Design review of the part built by this model. Coordinates are the model's own, in mm. A direction names the side the tool comes from. Give positions to 0.01 mm unless a question says otherwise; leave off trailing zeros. Loops run counter-clockwise (first coordinate to the right, second up) from the corner with the lowest first, then second, coordinate; pieces in that order, holes last. Notation, with made-up numbers: M -31,-3.5 L 19,-3.5 A23 cw 19,31.5 Z; hole C 88,-14.5 d3. An arc over 180 degrees is marked long. Use a Markdown table: item, result. Add a question column.
(1) Add section A-A, the plane y = 137. Give the boundary of the cut face in (x, z), then the cut area to 3 significant figures.
(2) For faces 1 (the face through (-0.86, 74.82, -3.874)), 2 (the face through (-6.35, -3, 0)), list the 3-axis set-ups (+Z, -Z, +X, -X, +Y, -Y) from which the entire face can be reached by the end or side of a thin tool; tool diameter is ignored.
(3) Insertion check: pin 1 Ø6 at (y, z) = (69, 4.5) entering from -X; pin 2 Ø1.5 at (x, y) = (-2, 24) entering from -Z; pin 3 Ø5 at (x, y) = (-2.5, 100.5) entering from -Z. Each pin has a flat end and moves straight along its axis. Give the tip position at first contact, or say it passes through.
(4) For probe 1 along Y at (x, z) = (2.5, 4.25); probe 2 along Z at (x, y) = (0, 46); probe 3 along X at (y, z) = (82, 1), list the stretches that pass through material, from the lowest coordinate up.
```python
from build123d import *

# Parameters (mm, degrees)
F2_R     = 3.96875
F3_DEPTH = 152.4
F5_DEPTH = 5.55625
F6_SIZE  = 0.635


# Not quite as in the source:
# - a length typed as a fraction of an inch, garbled in the dataset ("3 / 203.2 mm" for 3/8 in), is restored


with BuildPart() as f3:
    # F2 (on Front) → F3 (new body)
    with BuildSketch(Plane.XZ):
        Circle(F2_R)
    extrude(amount=-F3_DEPTH)

    # F4 (on Front) → F5 (join)
    with BuildSketch(Plane.XZ):
        Polygon((0, -7.3323484187), (6.35, -3.6661742094), (6.35, 3.6661742094), (0, 7.3323484187), (-6.35, 3.6661742094), (-6.35, -3.6661742094), align=None)
    extrude(amount=F5_DEPTH)

    # F6
    f6_edges = [f3.edges().sort_by_distance(p)[0] for p in [
        (-3.96875, 152.4, 0),
    ]]
    chamfer(f6_edges, length=F6_SIZE)

    # F7 (on Top) → F8 (revolve, cut)
    with BuildSketch(Plane.XY):
        Polygon((13.4339599431, -5.55625), (13.4339599431, -1.4663238199), (6.35, -5.55625), align=None)
    revolve(axis=Axis((0, -2.778125, 0), (0, -1, 0)), mode=Mode.SUBTRACT)


solid = f3.part
```
Established:
| question | item | result |
|---|---|---|
| 1 | outline | C 0,0 d7.94 |
| 1 | area | 49.5 mm^2 |
| 2 | face 1 | +Y |
| 2 | face 2 | +Z, -Z, -X, +Y, -Y |
| 3 | pin 1 | x = -3.67 |
| 3 | pin 2 | z = -3.77 |
| 3 | pin 3 | z = -3.97 |
| 4 | probe 1 | -5.56 to 0 |
| 4 | probe 2 | -3.97 to 3.97 |
| 4 | probe 3 | -3.84 to 3.84 |
